CAD build for the part. Positions are in the model's coordinates, mm. A direction names the side the tool comes from. Give positions to 0.01 mm unless a question says otherwise; leave off trailing zeros. Loops run counter-clockwise (first coordinate to the right, second up) from the corner with the lowest first, then second, coordinate; pieces in that order, holes last. Notation, with made-up numbers: (14, 11.5) - (46, 11.5) arc R12 ccw to (46, 30.5) - close; hole circle Ø3 at (11.5, -7). An arc over 180 degrees is marked (long way). Return JSON: item names as keys, results as strings.
from build123d import *

# Parameters (mm, degrees)
F0_W     = 50.8
F0_H     = 10.16
F1_DEPTH = 7.62
F2_DEPTH = 2.54


with BuildPart() as f1:
    # F0 (on Top) → F1 (new body)
    with BuildSketch(Plane.XY):
        with BuildLine():
            Line((0, 20.32), (-63.5, 20.32))
            Line((-63.5, 20.32), (-63.5, 0))
            Line((-63.5, 0), (-63.5, -18.967217))
            Line((-63.5, -18.967217), (-55.88, -18.967217))
            ThreePointArc((-55.88, -18.967217), (-50.8, -13.887217), (-45.72, -18.967217))
            Line((-45.72, -18.967217), (-43.18, -18.967217))
            ThreePointArc((-43.18, -18.967217), (-38.1, -13.887217), (-33.02, -18.967217))
            Line((-33.02, -18.967217), (33.02, -18.967217))
            ThreePointArc((33.02, -18.967217), (38.1, -13.887217), (43.18, -18.967217))
            Line((43.18, -18.967217), (45.72, -18.967217))
            ThreePointArc((45.72, -18.967217), (50.8, -13.887217), (55.88, -18.967217))
            Line((55.88, -18.967217), (63.5, -18.967217))
            Line((63.5, -18.967217), (63.5, 0))
            Line((63.5, 0), (63.5, 20.32))
            Line((63.5, 20.32), (0, 20.32))
        make_face()
        with Locations((0, -8.807217)):
            Rectangle(F0_W, F0_H, mode=Mode.SUBTRACT)
        Polygon((-1.463309, 4.427512), (-52.07, 0), (-52.955502, 10.121338), (-2.348812, 14.54885), align=None, mode=Mode.SUBTRACT)
        Polygon((2.348812, 14.54885), (52.955502, 10.121338), (52.07, 0), (1.463309, 4.427512), align=None, mode=Mode.SUBTRACT)
        with BuildLine():
            Line((-55.88, -18.967217), (-63.5, -18.967217))
            Line((-63.5, -18.967217), (-63.5, -30.48))
            Line((-63.5, -30.48), (0, -30.48))
            Line((0, -30.48), (63.5, -30.48))
            Line((63.5, -30.48), (63.5, -18.967217))
            Line((63.5, -18.967217), (55.88, -18.967217))
            ThreePointArc((55.88, -18.967217), (50.8, -24.047217), (45.72, -18.967217))
            Line((45.72, -18.967217), (43.18, -18.967217))
            ThreePointArc((43.18, -18.967217), (38.1, -24.047217), (33.02, -18.967217))
            Line((33.02, -18.967217), (-33.02, -18.967217))
            ThreePointArc((-33.02, -18.967217), (-38.1, -24.047217), (-43.18, -18.967217))
            Line((-43.18, -18.967217), (-45.72, -18.967217))
            ThreePointArc((-45.72, -18.967217), (-50.8, -24.047217), (-55.88, -18.967217))
        make_face()
    extrude(amount=F1_DEPTH)

    # F0 (on Top) → F2 (join)
    with BuildSketch(Plane.XY):
        with Locations((0, -8.807217)):
            Rectangle(F0_W, F0_H)
        Polygon((-52.955502, 10.121338), (-52.07, 0), (-1.463309, 4.427512), (-2.348812, 14.54885), align=None)
        Polygon((52.07, 0), (52.955502, 10.121338), (2.348812, 14.54885), (1.463309, 4.427512), align=None)
    extrude(amount=F2_DEPTH)


solid = f1.part
1. Drop flat-ended pins along their axis: P1, Ø3, axis at x = -0.5, y = -9.5, coming from the +Z side; P2, Ø1, axis at x = -37.5, y = -14.5, coming from the +Z side. Give the stop position or say it passes through.
Values follow:
{"P1": "stops at z = 2.54", "P2": "passes through"}
2. Cut at B-B, the plane x = -50.8. Write the cut outline in (y, z), plus the area to 3 significant figures.
Values follow:
{"outline": "(-30.48, 0) - (-24.05, 0) - (-24.05, 7.62) - (-30.48, 7.62) - close; (-13.89, 0) - (20.32, 0) - (20.32, 7.62) - (10.31, 7.62) - (10.31, 2.54) - (0.11, 2.54) - (0.11, 7.62) - (-13.89, 7.62) - close", "area": "258 mm²"}
3. Pull direction Y, two halves, no side cores. Call faces 3 (the face through (-1, -30.48, 4)), 4 (the face through (52.52, 5.13, 5.04)), 5 (the face through (-1, -5, 0)): +Y half, -Y half, draft (parallel to the pull), parting line (faces both ways), or undercut.
Values follow:
{"face 3": "-Y half", "face 4": "undercut", "face 5": "draft"}
4. Cut at A-A, the plane y = -10. Write the cut outline in (x, z), plus the area to 3 significant figures.
Values follow:
{"outline": "(-63.5, 0) - (63.5, 0) - (63.5, 7.62) - (25.4, 7.62) - (25.4, 2.54) - (-25.4, 2.54) - (-25.4, 7.62) - (-63.5, 7.62) - close", "area": "710 mm²"}
5. Cut at C-C, the plane z = 4.5. Write the cut outline in (x, y).
Values follow:
{"outline": "(-63.5, -30.48) - (63.5, -30.48) - (63.5, 20.32) - (-63.5, 20.32) - close; hole circle Ø10.16 at (-50.8, -18.97); hole (-52.96, 10.12) - (-52.07, 0) - (-1.46, 4.43) - (-2.35, 14.55) - close; hole circle Ø10.16 at (-38.1, -18.97); hole (-25.4, -13.89) - (25.4, -13.89) - (25.4, -3.73) - (-25.4, -3.73) - close; hole (1.46, 4.43) - (52.07, 0) - (52.96, 10.12) - (2.35, 14.55) - close; hole circle Ø10.16 at (38.1, -18.97); hole circle Ø10.16 at (50.8, -18.97)"}
6. Drill centre lines: probe 1 along Y at (x, z) = (-50.8, 3.75); probe 2 along Y at (x, z) = (38.1, 2.5); probe 3 along X at (y, z) = (-17.5, 6.5). Where is each one in solid material? Low to high.
Values follow:
{"probe 1": "y = -30.48 to -24.05, -13.89 to 0.11, 10.31 to 20.32", "probe 2": "y = -30.48 to -24.05, -13.89 to 20.32", "probe 3": "x = -63.5 to -55.66, -45.94 to -42.96, -33.24 to 33.24, 42.96 to 45.94, 55.66 to 63.5"}
7. Which spindle directions (+Z, -Z, +X, -X, +Y, -Y) get a long thin tool onto all of the face, cutting with end or side? Do faces 1 (the face through (27.121, 2.183, 5.044)), 2 (the face through (-63.5, -5, 4)). Say none if no direction does.
Values follow:
{"face 1": "+Z", "face 2": "+Z, -Z, -X, +Y, -Y"}
8. Cut at D-D, the plane x = -18. Write the cut outline in (y, z).
Values follow:
{"outline": "(-30.48, 0) - (20.32, 0) - (20.32, 7.62) - (13.18, 7.62) - (13.18, 2.54) - (2.98, 2.54) - (2.98, 7.62) - (-3.73, 7.62) - (-3.73, 2.54) - (-13.89, 2.54) - (-13.89, 7.62) - (-30.48, 7.62) - close"}
